Autodesk Inventor part; units mm, degrees
ref_plane "YZ Plane" through (0, 0, 0) normal (1, 0, 0) x (0, 1, 0)
ref_plane "XZ Plane" through (0, 0, 0) normal (0, 1, 0) x (-1, 0, 0)
ref_plane "XY Plane" through (0, 0, 0) normal (0, 0, 1) x (1, 0, 0)
sketch "Sketch1" plane through (0, 0, 0) normal (0, 1, 0) x (-1, 0, 0)
  line L0 (-49.6221, -50.9693) -> (50.3779, -50.9693)
  line L1 (50.3779, -50.9693) -> (50.3779, 49.0307)
  line L2 (50.3779, 49.0307) -> (-49.6221, 49.0307)
  line L3 (-49.6221, 49.0307) -> (-49.6221, -50.9693)
  line L4 (-17.8721, -0.5117) -> (18.6279, -0.5117)
  line L5 (18.6279, -0.5117) -> (18.6279, -50.9693)
  line L6 (18.6279, -50.9693) -> (-17.8721, -50.9693)
  line L7 (-17.8721, -50.9693) -> (-17.8721, -0.5117)
  line L8 (-49.6221, -18.7693) -> (50.3779, -18.7693)
  line L9 (50.3779, -18.7693) -> (50.3779, -50.9693)
  line L10 (50.3779, -50.9693) -> (-49.6221, -50.9693)
  line L11 (-49.6221, -50.9693) -> (-49.6221, -18.7693)
  line L12 (-49.6221, -18.7693) -> (50.3779, -18.7693)
  line L13 (50.3779, -18.7693) -> (50.3779, -14.7693)
  line L14 (50.3779, -14.7693) -> (-49.6221, -14.7693)
  line L15 (-49.6221, -14.7693) -> (-49.6221, -18.7693)
  line L16 (-49.6221, -34.8693) -> (50.3779, -34.8693)
  line L17 (-49.6221, -50.9693) -> (50.3779, -50.9693)
  line L18 (50.3779, -50.9693) -> (50.3779, -46.9693)
  line L19 (50.3779, -46.9693) -> (-49.6221, -46.9693)
  line L20 (-49.6221, -46.9693) -> (-49.6221, -50.9693)
  point P0 (0, 0)
  point P1 (0.3779, -50.9693)
  point P2 (0.3779, -50.9693)
  point P3 (0.3779, -50.9693)
  point P4 (-49.6221, -14.7693)
  point P5 (-17.8721, -14.7693)
  point P6 (-17.8721, -46.9693)
  point P7 (18.6279, -46.9693)
  point P8 (18.6279, -14.7693)
  dimension "d0" = 100
  dimension "d1" = 100
  dimension "d2" = 36.5
  dimension "d3" = 100
  dimension "d4" = 32.2
  dimension "d5" = 4
  dimension "d6" = 4
extrude "Extrusion1" add sketch "Sketch1" along normal blind 4 contours L7 L16 L5 L19 | L7 L8 L5 L16 | L7 L14 L5 L8 | L3 L2 L1 L14 L5 L4 L7 | L7 L4 L5 L14
sketch "Sketch2" plane through (17.8721, 0, -14.7693) normal (1, 0, 0) x (0, 0, -1)
  line L0 (0, 0) -> (32.2, 0)
  line L1 (32.2, 0) -> (32.2, 4)
  line L2 (0, 4) -> (32.2, 4)
  line L3 (0, 0) -> (0, 4)
  circle A0 centre (20.1, 13.6) radius 16.1
  line L4 (32.2, 0) -> (32.2, 4)
  circle A1 centre (20.1, 13.6) radius 15.4457
  point P0 (-14.7693, 0)
  point P1 (27.4219, 0)
extrude "Extrusion2" cut sketch "Sketch2" against normal through all contours A0 L1 L0 | L0 A1 L1 A0
sketch "Sketch3" plane through (0, 0, 0) normal (0, -1, 0) x (1, 0, 0)
  line L0 (-18.6279, -46.9693) -> (-18.6279, -42.1911)
  line L1 (17.8721, -46.9693) -> (-18.6279, -46.9693)
  line L2 (17.8721, -42.1911) -> (17.8721, -46.9693)
  line L3 (-18.6279, -42.1911) -> (17.8721, -42.1911)
  line L4 (-18.6279, -42.1911) -> (17.8721, -42.1911)
  line L5 (17.8721, -14.7693) -> (17.8721, -42.1911)
  line L6 (49.6221, -14.7693) -> (17.8721, -14.7693)
  line L7 (49.6221, 49.0307) -> (49.6221, -14.7693)
  line L8 (-50.3779, 49.0307) -> (49.6221, 49.0307)
  line L9 (-50.3779, -14.7693) -> (-50.3779, 49.0307)
  line L10 (-18.6279, -14.7693) -> (-50.3779, -14.7693)
  line L11 (-18.6279, -42.1911) -> (-18.6279, -14.7693)
  line L12 (17.8721, -46.9693) -> (-18.6279, -46.9693)
  line L13 (-18.6279, -42.1911) -> (17.8721, -42.1911)
  line L14 (2.6221, -34.1911) -> (-3.3779, -34.1911)
  line L15 (-3.3779, -34.1911) -> (-3.3779, -42.1911)
  line L16 (-3.3779, -42.1911) -> (2.6221, -42.1911)
  line L17 (2.6221, -42.1911) -> (2.6221, -34.1911)
  line L18 (2.6221, -42.1911) -> (-3.3779, -42.1911)
  line L19 (-3.3779, -42.1911) -> (-3.3779, -53.2472)
  line L20 (-3.3779, -53.2472) -> (2.6221, -53.2472)
  line L21 (2.6221, -53.2472) -> (2.6221, -42.1911)
  point P0 (0, 0)
  point P1 (-0.3779, -46.9693)
  point P2 (-0.3779, -42.1911)
  point P3 (-0.3779, -42.1911)
  dimension "d11" = 6
  dimension "d12" = 8
extrude "Extrusion3" cut sketch "Sketch3" against normal blind 2 contours L19 L3 L21 L1 | L1 L21 L20 L19 | L15 L14 L17 L3
sketch "Sketch4" plane through (0, 4, 0) normal (0, 1, 0) x (1, 0, 0)
  line L0 (49.6221, -49.0307) -> (49.6221, 14.7693)
  line L1 (49.6221, 14.7693) -> (17.8721, 14.7693)
  line L2 (17.8721, 14.7693) -> (17.8721, 46.9693)
  line L3 (17.8721, 46.9693) -> (-18.6279, 46.9693)
  line L4 (-18.6279, 46.9693) -> (-18.6279, 14.7693)
  line L5 (-18.6279, 14.7693) -> (-50.3779, 14.7693)
  line L6 (-50.3779, 14.7693) -> (-50.3779, -49.0307)
  line L7 (-50.3779, -49.0307) -> (49.6221, -49.0307)
  point P0 (0, 0)
extrude "Extrusion4" add sketch "Sketch4" along normal blind 1
sketch "Sketch5" plane through (17.8721, 0, -14.7693) normal (1, 0, 0) x (0, 0, -1)
  arc A0 (27.4219, 0) -> (32.2, 4) centre (20.1, 13.6) ccw
  arc A1 (27.4219, 0) -> (32.2, 4) centre (20.1, 13.6) ccw
  circle A2 centre (20.1, 13.6) radius 15.4457
  arc A3 (27.4219, 0) -> (32.2, 4) centre (20.1, 13.6) ccw
  line L0 (32.2, 4) -> (32.2, 5)
  line L1 (0, 5) -> (32.2, 5)
  line L2 (0, 0) -> (0, 5)
  line L3 (0, 0) -> (27.4219, 0)
  line L4 (32.2, 5) -> (32.93, 5)
  point P0 (-14.7693, 0)
  point P1 (32.2, 4)
extrude "Extrusion5" add sketch "Sketch5" against normal up to surface (36.5 mm away) contours L0 L4 A2
sketch "Sketch6" plane through (0, 2, 0) normal (0, -1, 0) x (1, 0, 0)
  line L0 (2.6221, -45.0678) -> (-3.3779, -45.0678)
  line L1 (2.6221, -34.1911) -> (2.6221, -45.0678)
  line L2 (-3.3779, -34.1911) -> (2.6221, -34.1911)
  line L3 (-3.3779, -45.0678) -> (-3.3779, -34.1911)
  line L4 (-3.3779, -34.1911) -> (2.6221, -34.1911)
  line L5 (-0.3779, -34.1911) -> (-0.3779, -35.8821)
  line L6 (-0.3779, -34.1911) -> (-0.3779, -36.935)
  circle A0 centre (-0.3779, -36.935) radius 1.5
  point P0 (0, 0)
  dimension "d19" = 3
extrude "Extrusion6" cut sketch "Sketch6" against normal blind 10 contours A0
sketch "Sketch7" plane through (49.6221, 0, 49.0307) normal (1, 0, 0) x (0, 0, -1)
  circle A0 centre (83.9, 13.6) radius 16.1
  line L0 (0, 0) -> (63.8, 0)
  line L1 (63.8, 0) -> (63.8, 5)
  line L2 (0, 5) -> (63.8, 5)
  line L3 (0, 0) -> (0, 5)
  arc A1 (91.2219, 0) -> (96.73, 5) centre (83.9, 13.6) ccw
  line L4 (63.8, 5) -> (96.73, 5)
  line L5 (63.8, 0) -> (63.8, 5)
  line L6 (63.8, 0) -> (91.2219, 0)
  line L7 (0, 0) -> (63.8, 0)
  line L8 (0, 0) -> (0, -14.6713)
  line L9 (83.9, -2.5) -> (-11.8385, -2.5)
  line L10 (91.2219, 0) -> (63.8, 0)
  line L11 (3.6899, -2.5) -> (17.1336, 5)
  line L12 (0, 5) -> (63.8, 5)
  line L13 (17.1336, 5) -> (28.2336, 16.1)
  line L14 (17.1336, 5) -> (32.8313, 5) construction
  line L15 (28.2336, 16.1) -> (29.6478, 14.6857)
  line L16 (29.6478, 14.6857) -> (19.962, 5)
  line L17 (83.9, 29.7) -> (9.0674, 29.7)
  line L18 (29.6478, 14.6857) -> (44.662, 29.7)
  line L19 (63.8, 5) -> (96.73, 5)
  circle A2 centre (83.9, 13.6) radius 21.8625
  line L20 (17.1336, 5) -> (1.0083, -2.5)
  point P0 (49.0307, 0)
  point P1 (6.3834, 0)
  dimension "d22" = 45
  dimension "d23" = 2
extrude "Extrusion7" cut sketch "Sketch7" against normal through all contours L20 L0 L3 L2
sketch "Sketch8" plane through (49.6221, 0, -14.7693) normal (1, 0, 0) x (0, 0, -1)
  line L0 (-46.6664, 5) -> (-57.4166, 0)
  line L1 (-57.4166, 0) -> (0, 0)
  line L2 (0, 0) -> (0, 5)
  line L3 (-46.6664, 5) -> (0, 5)
  line L4 (0, 5) -> (-46.6664, 5)
  line L5 (-45.5728, 5) -> (-39.1497, 11.4231)
  line L6 (-45.5728, 5) -> (-36.4892, 5) construction
  line L7 (-39.1497, 11.4231) -> (-37.7355, 10.0089)
  line L8 (-37.7355, 10.0089) -> (-42.7444, 5)
  line L9 (-42.7444, 5) -> (-5.7272, 42.0172)
  circle A0 centre (20.1, 13.6) radius 16.1
  line L10 (20.1, 29.7) -> (-35.8827, 29.7)
  line L11 (32.93, 5) -> (0, 5)
  circle A1 centre (20.1, 13.6) radius 21.8625
  point P0 (-14.7693, 0)
  point P1 (5.3095, 29.7)
  point P2 (-18.0444, 29.7)
  dimension "d26" = 45
  dimension "d27" = 2
extrude "Extrusion8" add sketch "Sketch8" against normal blind 6 contours L8 L9 L10 A1 L3
sketch "Sketch9" plane through (-50.3779, 0, -14.7693) normal (-1, 0, 0) x (0, 0, 1)
  line L0 (57.4166, 0) -> (46.6664, 5)
  line L1 (0, 5) -> (46.6664, 5)
  line L2 (0, 0) -> (0, 5)
  line L3 (0, 0) -> (57.4166, 0)
  line L4 (18.0444, 29.7) -> (-5.3095, 29.7)
  arc A0 (0, 5) -> (-5.3095, 29.7) centre (-20.1, 13.6) ccw
  line L5 (42.7444, 5) -> (0, 5)
  line L6 (42.7444, 5) -> (18.0444, 29.7)
  point P0 (14.7693, 0)
extrude "Extrusion9" add sketch "Sketch9" against normal blind 6 contours L1 A0 L4 L6
sketch "Sketch10" plane through (0, 5, 0) normal (0, 1, 0) x (1, 0, 0)
  line L0 (-44.3779, -27.9751) -> (-50.3779, -27.9751)
  line L1 (-50.3779, -27.9751) -> (-50.3779, -31.8971)
  line L2 (-50.3779, -31.8971) -> (49.6221, -31.8971)
  line L3 (49.6221, -31.8971) -> (49.6221, -27.9751)
  line L4 (49.6221, -27.9751) -> (43.6221, -27.9751)
  line L5 (43.6221, -27.9751) -> (43.6221, 14.7693)
  line L6 (43.6221, 14.7693) -> (17.8721, 14.7693)
  line L7 (17.8721, 14.7693) -> (17.8721, 47.6993)
  line L8 (17.8721, 47.6993) -> (-18.6279, 47.6993)
  line L9 (-18.6279, 47.6993) -> (-18.6279, 14.7693)
  line L10 (-18.6279, 14.7693) -> (-44.3779, 14.7693)
  line L11 (-44.3779, 14.7693) -> (-44.3779, -27.9751)
  circle A0 centre (-0.3779, 36.935) radius 1.5
  line L12 (43.6221, -27.9751) -> (43.6221, 14.7693)
  line L13 (17.8721, 14.7693) -> (43.6221, 14.7693)
  line L14 (43.6221, 14.7693) -> (43.6221, 11.7693)
  line L15 (43.6221, 11.7693) -> (17.8721, 11.7693)
  line L16 (17.8721, 11.7693) -> (17.8721, 14.7693)
  line L17 (-44.3779, 14.7693) -> (-44.3779, -27.9751)
  line L18 (-18.6279, 14.7693) -> (-44.3779, 14.7693)
  line L19 (-44.3779, 14.7693) -> (-44.3779, 11.7693)
  line L20 (-44.3779, 11.7693) -> (-18.6279, 11.7693)
  line L21 (-18.6279, 11.7693) -> (-18.6279, 14.7693)
  point P0 (0, 0)
  dimension "d32" = 3
  dimension "d33" = 3
extrude "Extrusion10" add sketch "Sketch10" along normal blind 8 contours L11 L10 L21 L20 | L15 L16 L6 L5
sketch "Sketch11" plane through (-50.3779, 0, -14.7693) normal (-1, 0, 0) x (0, 0, 1)
  arc A0 (0, 5) -> (1.7543, 13) centre (-20.1, 13.6) ccw
  line L0 (0, 13) -> (1.7543, 13)
  line L1 (0, 5) -> (0, 13)
  point P0 (14.7693, 0)
extrude "Extrusion11" cut sketch "Sketch11" against normal through all
sketch "Sketch12" plane through (0, 0, 0) normal (0, -1, 0) x (1, 0, 0)
  line L0 (49.6221, 42.6473) -> (-50.3779, 42.6473)
  line L1 (-50.3779, -14.7693) -> (-50.3779, 42.6473)
  line L2 (-18.6279, -14.7693) -> (-50.3779, -14.7693)
  line L3 (-18.6279, -42.1911) -> (-18.6279, -14.7693)
  line L4 (-18.6279, -42.1911) -> (-3.3779, -42.1911)
  line L5 (-3.3779, -42.1911) -> (-3.3779, -34.1911)
  line L6 (-3.3779, -34.1911) -> (2.6221, -34.1911)
  line L7 (2.6221, -34.1911) -> (2.6221, -42.1911)
  line L8 (2.6221, -42.1911) -> (17.8721, -42.1911)
  line L9 (17.8721, -14.7693) -> (17.8721, -42.1911)
  line L10 (49.6221, -14.7693) -> (17.8721, -14.7693)
  line L11 (49.6221, 42.6473) -> (49.6221, -14.7693)
  circle A0 centre (-0.3779, -36.935) radius 1.5
  line L12 (17.8721, -14.7693) -> (17.8721, -47.6993)
  line L13 (17.8721, -47.6993) -> (-18.6279, -47.6993)
  line L14 (-18.6279, -47.6993) -> (-18.6279, -14.7693)
  line L15 (-18.6279, -14.7693) -> (-18.6279, -11.7693)
  line L16 (-18.6279, -11.7693) -> (-44.3779, -11.7693)
  line L17 (-44.3779, -11.7693) -> (-44.3779, 27.9751)
  line L18 (-44.3779, 27.9751) -> (-50.3779, 27.9751)
  line L19 (-50.3779, 27.9751) -> (-50.3779, 31.8971)
  line L20 (-50.3779, 31.8971) -> (49.6221, 31.8971)
  line L21 (49.6221, 31.8971) -> (49.6221, 27.9751)
  line L22 (49.6221, 27.9751) -> (43.6221, 27.9751)
  line L23 (43.6221, 27.9751) -> (43.6221, -11.7693)
  line L24 (43.6221, -11.7693) -> (17.8721, -11.7693)
  line L25 (17.8721, -11.7693) -> (17.8721, -14.7693)
  line L26 (-44.3779, -11.7693) -> (-44.3779, 27.9751)
  line L27 (-44.3779, 27.9751) -> (-42.3779, 27.9751)
  line L28 (-42.3779, 27.9751) -> (-36.3779, 27.9751)
  line L29 (-36.3779, 27.9751) -> (-36.3779, 19.9751)
  line L30 (-36.3779, 19.9751) -> (-42.3779, 19.9751)
  line L31 (-42.3779, 19.9751) -> (-42.3779, 27.9751)
  line L32 (43.6221, 27.9751) -> (43.6221, -11.7693)
  line L33 (43.6221, 27.9751) -> (41.6221, 27.9751)
  line L34 (41.6221, 27.9751) -> (35.6221, 27.9751)
  line L35 (35.6221, 27.9751) -> (35.6221, 19.9751)
  line L36 (35.6221, 19.9751) -> (41.6221, 19.9751)
  line L37 (41.6221, 19.9751) -> (41.6221, 27.9751)
  point P0 (0, 0)
  dimension "d38" = 2
  dimension "d39" = 6
  dimension "d40" = 8
  dimension "d41" = 2
  dimension "d42" = 6
extrude "Extrusion12" cut sketch "Sketch12" against normal blind 2 contours L28 L29 L30 L31 | L37 L36 L35 L34
sketch "Sketch13" plane through (0, 2, 0) normal (0, -1, 0) x (1, 0, 0)
  line L0 (35.6221, 19.9751) -> (35.6221, 27.9751)
  line L1 (41.6221, 19.9751) -> (35.6221, 19.9751)
  line L2 (41.6221, 27.9751) -> (41.6221, 19.9751)
  line L3 (35.6221, 27.9751) -> (41.6221, 27.9751)
  line L4 (-36.3779, 19.9751) -> (-42.3779, 19.9751)
  line L5 (-36.3779, 27.9751) -> (-36.3779, 19.9751)
  line L6 (-42.3779, 27.9751) -> (-36.3779, 27.9751)
  line L7 (-42.3779, 19.9751) -> (-42.3779, 27.9751)
  line L8 (-36.3779, 27.9751) -> (-36.3779, 19.9751)
  line L9 (-42.3779, 19.9751) -> (-36.3779, 19.9751)
  line L10 (-36.3779, 19.9751) -> (-36.3779, 21.9751)
  line L11 (-36.3779, 21.9751) -> (-42.3779, 21.9751)
  line L12 (-42.3779, 21.9751) -> (-42.3779, 19.9751)
  line L13 (41.6221, 27.9751) -> (41.6221, 19.9751)
  line L14 (35.6221, 19.9751) -> (35.6221, 27.9751)
  line L15 (41.6221, 19.9751) -> (35.6221, 19.9751)
  line L16 (35.6221, 19.9751) -> (35.6221, 21.9751)
  line L17 (35.6221, 21.9751) -> (41.6221, 21.9751)
  line L18 (41.6221, 21.9751) -> (41.6221, 19.9751)
  point P0 (0, 0)
  dimension "d45" = 2
extrude "Extrusion13" cut sketch "Sketch13" against normal through all contours L0 L17 L2 L1 | L4 L7 L11 L5
properties part number "dół"
CAD build for the part. Positions are in the model's coordinates, mm. A direction names the side the tool comes from. Give positions to 0.01 mm unless a question says otherwise; leave off trailing zeros. Loops run counter-clockwise (first coordinate to the right, second up) from the corner with the lowest first, then second, coordinate; pieces in that order, holes last. Notation, with made-up numbers: M 85,78.25 L 139,78.25 A6 ccw 139,87.25 Z; hole C 20,75.5 d4. An arc over 180 degrees is marked long. Answer in a Markdown table with one row per item. Add a question column.
Item 1: Band-saw the part on A-A on z = 2. Give the cut face in (x, y), then the cut area to 3 significant figures.
Item 2: Tool access for faces 5 (the face through (17.872, 8, -13)), 6 (the face through (-39, 2, 19.975)), 7 (the face through (34, 2, -14.769)), 8 (the face through (-34, 2, -14.769)), 9 (the face through (41.622, 1, 23)): list every direction of +Z, -Z, +X, -X, +Y, -Y with a clear straight run to the whole face (end or side of a thin tool).
Item 3: Band-saw the part on B-B on y = 21.75. Give the cut face in (x, z).
Item 4: Band-saw the part on D-D on y = 3.75. Give the cut face in (x, z) (3 decimals).
Item 5: Band-saw the part on C-C on x = -25. Give the cut face in (y, z) (3 decimals), then the cut area to 3 significant figures.
Item 6: Mould opens along Y. For faces 1 (the face through (-31.683, 8.861, -13.527)), 2 (the face through (46.664, 18.379, -13.535)), 3 (the face through (-47.42, 18.01, -13.456)), 4 (the face through (39, 3, 21.975)) say: +Y half, -Y half, draft (parallel to the pull), parting line (faces both ways), or undercut.
Item 7: Drop flat-ended pins along their axis: P1, Ø1.8, axis at x = 38, z = 25, coming from the -Y side; P2, Ø0.6, axis at x = -35.5, z = -12.5, coming from the +Y side; P3, Ø5.5, axis at x = 27.5, y = 2, coming from the -Z side. Give the stop position or say it passes through.
Item 8: Probe probe 1 along X at (y, z) = (24, -13); probe 2 along Y at (x, z) = (9.5, 20); probe 3 along X at (y, z) = (3, -38). List the from-to ranges inside material, lowest first.
Reply:
| question | item | result |
|---|---|---|
| 1 | outline | M -50.38,0 L 49.62,0 L 49.62,29.7 L 43.62,29.7 L 43.62,5 L -44.38,5 L -44.38,29.7 L -50.38,29.7 Z |
| 1 | area | 796 mm^2 |
| 2 | face 5 | +Z, -Z, +Y |
| 2 | face 6 | +Y, -Y |
| 2 | face 7 | -Z, +X, -Y |
| 2 | face 8 | -Z, -X, -Y |
| 2 | face 9 | -Y |
| 3 | outline | M -50.38,-14.58 L -44.38,-14.58 L -44.38,11.23 L -50.38,11.23 Z; M 43.62,-14.58 L 49.62,-14.58 L 49.62,11.23 L 43.62,11.23 Z |
| 4 | outline | M -50.378,-14.769 L -18.628,-14.769 L -18.628,-46.767 L 17.872,-46.767 L 17.872,-14.769 L 49.622,-14.769 L 49.622,34.585 L -50.378,34.585 Z; hole M -42.378,19.975 L -36.378,19.975 L -36.378,21.975 L -42.378,21.975 Z; hole C -0.378,-36.935 d3; hole M 35.622,19.975 L 41.622,19.975 L 41.622,21.975 L 35.622,21.975 Z |
| 5 | outline | M 0,-14.769 L 5,-14.769 A21.863 cw 13,-13.015 L 13,-11.769 L 5,-11.769 L 5,31.897 L 0,42.647 Z |
| 5 | area | 275 mm^2 |
| 6 | face 1 | +Y half |
| 6 | face 2 | undercut |
| 6 | face 3 | undercut |
| 6 | face 4 | draft |
| 7 | P1 | stops at y = 2 |
| 7 | P2 | stops at y = 13 |
| 7 | P3 | stops at z = -14.77 |
| 8 | probe 1 | x = -50.38 to -44.38, 43.62 to 49.62 |
| 8 | probe 2 | y = 0 to 5 |
| 8 | probe 3 | x = -18.63 to -1.43, 0.68 to 17.87 |
